```python
from build123d import *

# Parameters (mm, degrees)
SKETCH1_W                               = 200
SKETCH1_H                               = 200
BOSS_EXTRUDE1_DEPTH                     = 10
SKETCH2_R                               = 80
BOSS_EXTRUDE2_DEPTH                     = 100
SKETCH3_R                               = 50
CUT_EXTRUDE1_DEPTH                      = 100
SKETCH4_R                               = 70
CUT_EXTRUDE2_DEPTH                      = 10
CBORE_FOR_M8_HEX_HEAD_BOLT1_D           = 9
CBORE_FOR_M8_HEX_HEAD_BOLT1_CBORE_D     = 18.01
CBORE_FOR_M8_HEX_HEAD_BOLT1_CBORE_DEPTH = 5.68


with BuildPart() as part:
    # Sketch1 → Boss-Extrude1 (new body)
    with BuildSketch(Plane(origin=(0, 0, 0), x_dir=(1, 0, 0), z_dir=(0, 1, 0))):
        Rectangle(SKETCH1_W, SKETCH1_H)
    extrude(amount=BOSS_EXTRUDE1_DEPTH)

    # Sketch2 → Boss-Extrude2 (add)
    with BuildSketch(Plane(origin=(0, 10, 0), x_dir=(1, 0, 0), z_dir=(0, 1, 0))):
        Circle(SKETCH2_R)
    extrude(amount=BOSS_EXTRUDE2_DEPTH)

    # Sketch3 → Cut-Extrude1 (cut)
    with BuildSketch(Plane(origin=(0, 110, 0), x_dir=(1, 0, 0), z_dir=(0, 1, 0))):
        Circle(SKETCH3_R)
    extrude(amount=-CUT_EXTRUDE1_DEPTH, mode=Mode.SUBTRACT)

    # Sketch4 → Cut-Extrude2 (cut)
    with BuildSketch(Plane(origin=(0, 110, 0), x_dir=(1, 0, 0), z_dir=(0, 1, 0))):
        Circle(SKETCH4_R)
    extrude(amount=-CUT_EXTRUDE2_DEPTH, mode=Mode.SUBTRACT)

    # CBORE for M8 Hex Head Bolt1 (through all)
    with Locations(Plane(origin=(80, 10, -80), x_dir=(0, 0, 1), z_dir=(0, 1, 0))):
        with Locations((0, 0), (0, -160), (160, 0), (160, -160)):
            CounterBoreHole(CBORE_FOR_M8_HEX_HEAD_BOLT1_D / 2, CBORE_FOR_M8_HEX_HEAD_BOLT1_CBORE_D / 2, CBORE_FOR_M8_HEX_HEAD_BOLT1_CBORE_DEPTH)


solid = part.part
```
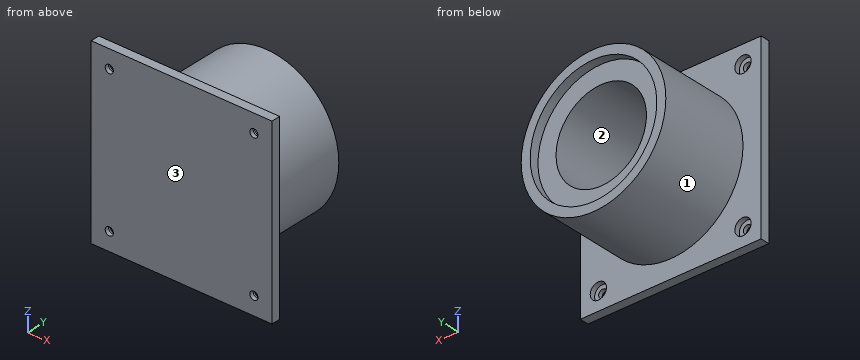
Geometry: final body of the model. Coordinates: model frame, mm. Face numbers are marked on the shaded views. Round coordinates to 2 decimals unless told otherwise and drop trailing zeros. Write each loop counter-clockwise with the first axis right and the second up, starting at its lowest first coordinate (ties: lowest second). Pieces come first, ordered by that corner, then holes.
Item 1: Section query A-A (z = -29.5). Return loops of the section in (x, y).
Item 2: Section query B-B (x = 24). Return loops of the section in (y, z), plus the area to 3 significant figures.
Item 3: Pin query (flat end, axial travel): P1, Ø2, axis at x = 10, z = 0.5, coming from the +Y side; P2, Ø4, axis at x = -8.5, z = -11.5, coming from the -Y side; P3, Ø6, axis at y = 71, z = -75, coming from the -X side; P4, Ø1, axis at x = 68, y = 65, coming from the +Z side. Return the tip coordinate at first contact, or that it passes through.
Item 4: Material intervals for L1, parallel to X at y = 1.4, z = 80; L2, parallel to X at y = 6.45, z = 80 (3 decimals); L3, parallel to X at y = 76.5, z = 0, sorted ascending.
Item 5: Mould query, pull axis X, two halves, no side actions, for the marked faces 1, 2 and 3. Classes: +X half, -X half, draft (parallel to the pull), parting line (faces both ways), or undercut.
Item 6: Section query C-C (y = 68). Return loops of the section in (x, z), plus the area to 3 significant figures.
Completed:
1. outline: (-100, 0) - (100, 0) - (100, 10) - (74.36, 10) - (74.36, 110) - (63.48, 110) - (63.48, 100) - (40.37, 100) - (40.37, 10) - (-40.37, 10) - (-40.37, 100) - (-63.48, 100) - (-63.48, 110) - (-74.36, 110) - (-74.36, 10) - (-100, 10) - close
2. outline: (0, -100) - (10, -100) - (10, -76.32) - (110, -76.32) - (110, -65.76) - (100, -65.76) - (100, -43.86) - (10, -43.86) - (10, 43.86) - (100, 43.86) - (100, 65.76) - (110, 65.76) - (110, 76.32) - (10, 76.32) - (10, 100) - (0, 100) - close
2. area: 8,050 mm2
3. P1: stops at y = 10
3. P2: stops at y = 0
3. P3: stops at x = -34.87
3. P4: stops at z = 42.94
4. L1: x = -100 to -84.5, -75.5 to 75.5, 84.5 to 100
4. L2: x = -100 to -89.005, -70.995 to 70.995, 89.005 to 100
4. L3: x = -80 to -50, 50 to 80
5. face 1: parting line
5. face 2: undercut
5. face 3: draft
6. outline: circle Ø160 at (0, 0); hole circle Ø100 at (0, 0)
6. area: 12,300 mm2
